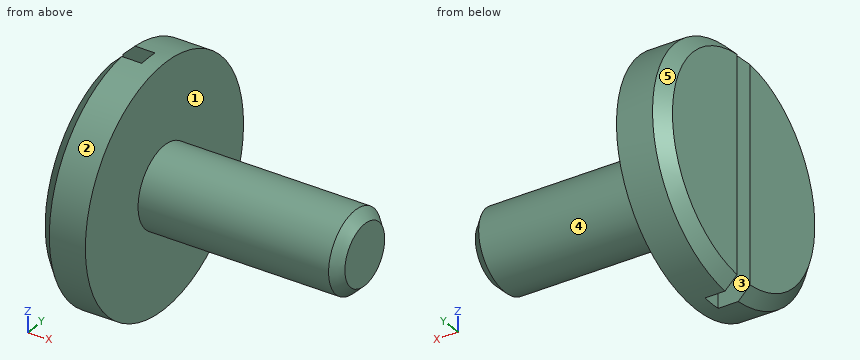
Autodesk Inventor part; units mm, degrees
ref_plane "Work Plane1" through (2.5, 0, 0) normal (0, 0, -1) x (1, 0, 0)
ref_plane "YZ Plane" through (0, 0, 0) normal (1, 0, 0) x (0, 1, 0)
ref_plane "XZ Plane" through (0, 0, 0) normal (0, 1, 0) x (-1, 0, 0)
sketch "Sketch1" plane through (0, 0, 0) normal (0, 0, 1) x (1, 0, 0)
  line L0 (-1.2, 0) -> (5, 0)
  line L1 (5, 0) -> (5, 1)
  line L2 (5, 1) -> (0, 1)
  line L3 (0, 1) -> (0, 3)
  line L4 (0, 3) -> (-1.2, 3)
  line L5 (-2.44, 0) -> (6.24, 0)
  line L6 (-1.2, 0) -> (-1.2, 3)
  line L7 (0, -0.6) -> (0, 3.6)
  dimension "d0" = 5
  dimension "d1" = 2
  dimension "d2" = 6
  dimension "d15" = 1.2
revolve "Body" add sketch "Sketch1" angle 360 about axis through (-1.2, 0, 0) along (1, 0, 0)
sketch "Sketch2" plane through (-1.2, 0, 0) normal (-1, 0, 0) x (0, 0, 1)
  circle A0 centre (0, 0) radius 3
  line L0 (0, -4.2) -> (0, 4.2)
  line L1 (-4.2, 0) -> (4.2, 0)
  line L2 (-3, 0.25) -> (3, 0.25)
  line L3 (3, 0.25) -> (3, -0.25)
  line L4 (3, -0.25) -> (-3, -0.25)
  line L5 (-3, -0.25) -> (-3, 0.25)
  line L6 (-3, 0) -> (3, 0) construction
  line L7 (0, 0.25) -> (0, -0.25) construction
  dimension "d10" = 0.5
extrude "Slot" cut sketch "Sketch2" against normal blind 0.8 contours L1 L0 L2 A0 | L3 L4 A0 | A0 L4 L0 L1 | A0 L2 L3 | L1 A0 L2 L0 | L0 L4 A0 L1 | L5 L2 A0 | A0 L4 L5
chamfer "Chamfer1" distance 0.3 angle 45 3 edges at (-1.2, -3, 0) (-1.2, 2.2079, 2.031) (-1.2, 2.2079, -2.031) measured on face at (-0.5333, -0.7686, -2.8999)
thread "Thread"
chamfer "Chamfer2" distance 0.2454 distance2 0.2454 1 edges at (5, -1, 0) measured on face at (5, 0.5392, -0.3309)
ref_plane "Work Plane1" through (2.5, 0, 0) normal (0, 0, -1) x (1, 0, 0)
equation "\"d0\" = NLG"
equation "\"d1\" = NND"
equation "\"d2\" = KOD"
equation "\"d15\" = KOH"
equation "\"d10\" = SBR"
equation "\"d11\" = STI"
equation "\"d13\" = PHH"
equation "\"d23\" = PHH"
equation "\"d3\" = GEL"
equation "\"d5\" = -0.5 * GD1 + 0.5 * NND"
equation "\"d6\" = GUL"
equation "\"NND\" = 2"
equation "\"NLG\" = 5"
equation "\"GEL\" = NLG - 2 * PTC"
equation "\"KOD\" = 6"
equation "\"KOH\" = 1.2"
equation "\"GUL\" = 0.61345 * PTC"
equation "\"PHH\" = 0.3"
equation "\"SBR\" = 0.5"
equation "\"STI\" = 0.8"
equation "\"GD1\" = THREADDIA - 1.2269 * PTC"
equation "\"THREADDIA\" = 2"
equation "\"TOA\" = 30deg"
equation "\"PTC\" = 0.4"
equation "\"GAL\" = 0.61345 * PTC"
properties part number "DIN 921 - M2 x 5" material "Steel, Mild"
Source: CAD feature listing. Evaluate the final solid. Frame: model axes, mm. Face numbers are marked on the shaded views. A direction names the side the tool comes from. Round coordinates to 2 decimals unless told otherwise and drop trailing zeros. Write each loop counter-clockwise with the first axis right and the second up, starting at its lowest first coordinate (ties: lowest second). Pieces come first, ordered by that corner, then holes. Notation, with made-up numbers: M 39,36 L 84,36 A24 cw 84,52 Z; hole C -37,-7 d8. An arc over 180 degrees is marked long. One line per item, written item: value. Start each with the question number.
Item 1: Section query A-A (z = 0). Return the cut outline in (x, y), plus the area to 3 significant figures.
Item 2: Set-up query: the marked faces 1 and 2. Return all of +Z, -Z, +X, -X, +Y, -Y with unobstructed straight access to the full face (end or side cutting, diameter ignored); none if empty.
Item 3: Pin query (flat end, axial travel): pin 1 (1.5 mm diameter, centred on x = 4, z = -0.5, fed in from +Y); pin 2 (0.9 mm diameter, centred on x = -0.5, z = -1, fed in from +Y). Return the tip coordinate at first contact, or that it passes through.
Item 4: Section query C-C (x = 4.25). Return the cut outline in (y, z).
Item 5: Ray query, L1, parallel to X at y = 1.5, z = -2; L2, parallel to X at y = -1.5, z = 2.5; L3, parallel to Z at x = 1, y = -0.25. Return the intervals inside material, ascending. Write a range as from..to.
Item 6: Section query B-B (y = 0). Return the cut outline in (x, z), plus the area to 3 significant figures.
Item 7: Mould query, pull axis Y, two halves, no side actions, for the marked faces 3, 4 and 5. Classes: pulls with the +Y half, pulls with the -Y half, needs draft (parallel to the pull), parting line crosses it, or undercut.
Result set:
1. outline: M -1.2,-2.7 L -0.9,-3 L 0,-3 L 0,-1 L 4.75,-1 L 5,-0.75 L 5,0.75 L 4.75,1 L 0,1 L 0,3 L -0.9,3 L -1.2,2.7 L -1.2,0.25 L -0.4,0.25 L -0.4,-0.25 L -1.2,-0.25 Z
1. area: 16.6 mm²
2. face 1: +X
2. face 2: +X, -X
3. pin 1: stops at y = 1
3. pin 2: stops at y = 2.95
4. outline: C 0,0 d2
5. L1: x = -1.2..0
5. L2: x = -0.98..0
5. L3: z = -0.97..0.97
6. outline: M -0.4,-3 L 0,-3 L 0,-1 L 4.75,-1 L 5,-0.75 L 5,0.75 L 4.75,1 L 0,1 L 0,3 L -0.4,3 Z
6. area: 12.3 mm²
7. face 3: undercut
7. face 4: parting line crosses it
7. face 5: pulls with the +Y half
